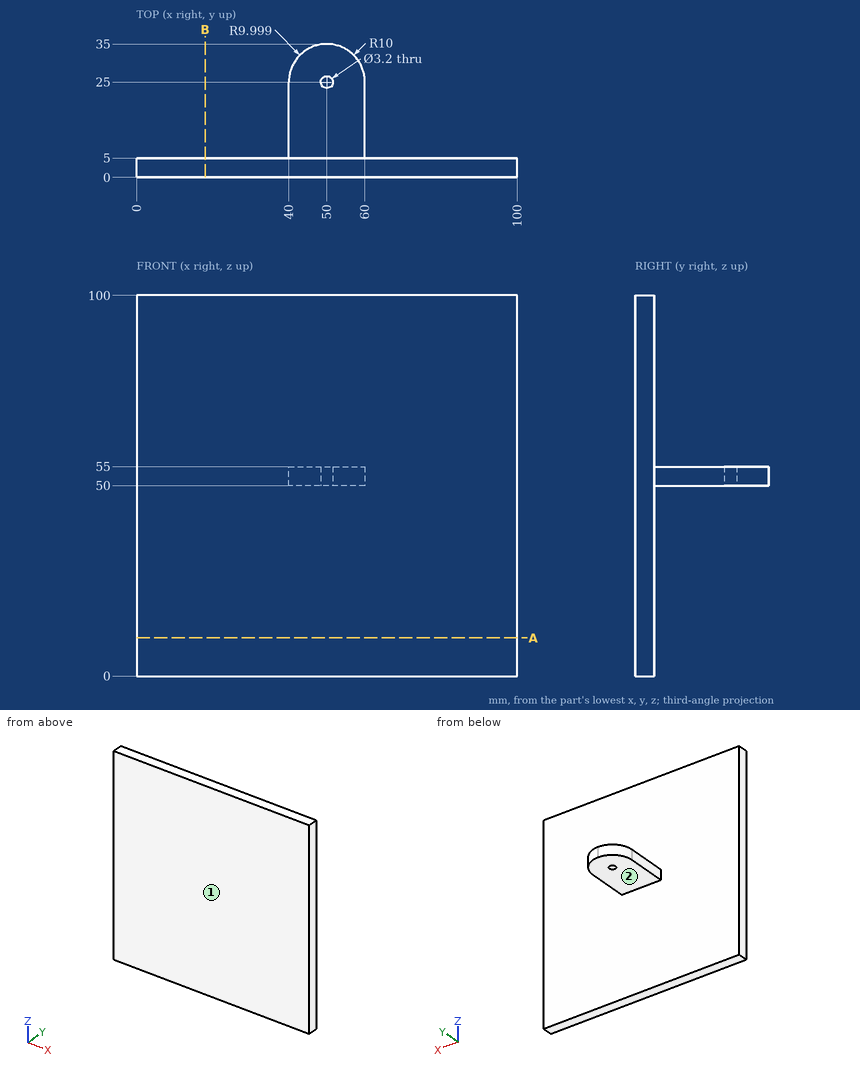
Check sheet for the drawn part. Datum: minimum x, y, z corner. Units: mm. A direction names the side the tool comes from. Give positions to 0.01 mm unless a question says otherwise; leave off trailing zeros. Order: outer loops, then holes, each group sorted by start corner. A loop starts at its lowest first (then second) coordinate and runs counter-clockwise, first axis right, second up. Notation, with made-up numbers: (11.5, 30.25) -> (42.5, 30.25) arc R24 cw to (42.5, 47.25) -> close; hole circle Ø4 at (64, 42). An arc over 180 degrees is marked (long way). Use a Markdown table: item, result.
1) Section check A-A, the plane z = 10. Record the boundary of the cut face in (x, y), then the cut area to 3 significant figures.
Results:
| item | result |
|---|---|
| outline | (0, 0) -> (100, 0) -> (100, 5) -> (0, 5) -> close |
| area | 500 mm² |
2) Section check B-B, the plane x = 18. Record the boundary of the cut face in (y, z).
Results:
| item | result |
|---|---|
| outline | (0, 0) -> (5, 0) -> (5, 100) -> (0, 100) -> close |
3) Depth check by flat-ended pin: pin 1 Ø2.5 at (y, z) = (12, 53.5) entering from -X; pin 2 Ø5 at (x, y) = (50, 25) entering from -Z; pin 3 Ø1.5 at (y, z) = (16.5, 53.5) entering from +X; pin 4 Ø8 at (x, z) = (87, 33.5) entering from -Y. Enter the tip coordinate at first touch or a pass-through.
Results:
| item | result |
|---|---|
| pin 1 | x = 40 |
| pin 2 | z = 50 |
| pin 3 | x = 60 |
| pin 4 | y = 0 |
4) Material ranges on probe 1 along X at (y, z) = (25, 51.7); probe 2 along Y at (x, z) = (50, 53); probe 3 along Y at (x, z) = (86.5, 41), recorded low to high.
Results:
| item | result |
|---|---|
| probe 1 | 40 to 48.4, 51.6 to 60 |
| probe 2 | 0 to 23.4, 26.6 to 35 |
| probe 3 | 0 to 5 |
5) Tool access check on the marked faces 1 and 2. Record the directions out of +Z, -Z, +X, -X, +Y, -Y that give a thin tool (end or side, any length) a straight path to the whole face; none if there is none.
Results:
| item | result |
|---|---|
| face 1 | +Z, -Z, +X, -X, -Y |
| face 2 | -Z, +X, -X, +Y |
